from build123d import *

# Parameters (mm, degrees)
F0_W        = 40.3080582619
F0_H        = 5.9715644456
F1_DEPTH    = 537
F3_DEPTH    = 1017
F5_DEPTH    = 5
F6_T1_DEPTH = 716.1336390313


# Not quite as in the source:
# - a fillet or chamfer that OpenCascade refuses, or shapes differently, is made with other operations: its cross-section is extruded or revolved along the edge and cut away or added


with BuildPart() as f1:
    # F0 (on Top) → F1 (new body)
    with BuildSketch(Plane.XY):
        Rectangle(F0_W, F0_H)
    extrude(amount=F1_DEPTH)

    # F2 (on Top) → F3 (join)
    with BuildSketch(Plane.XY):
        Polygon((6.5744029718, -8.407556447), (10.5938451005, -1.2962352533), (8.407556447, 6.5744029718), (1.2962352533, 10.5938451005), (-6.5744029718, 8.407556447), (-10.5938451005, 1.2962352533), (-8.407556447, -6.5744029718), (-1.2962352533, -10.5938451005), align=None)
    extrude(amount=-F3_DEPTH)

    # F4 (on Top) → F5 (join)
    with BuildSketch(Plane.XY):
        Polygon((31.1715127681, -0.1368859226), (15.7043030704, 26.9268789703), (-15.4672096977, 27.0637648929), (-31.1715127681, 0.1368859226), (-15.7043030704, -26.9268789703), (15.4672096977, -27.0637648929), align=None)
    extrude(amount=F5_DEPTH)

    # F6: fillet of radius 270.3919189858 on 1 edges, made by hand

    # F6_s2 → F6_t1 (cut)
    with BuildSketch(Plane.XZ.offset(-358.0668195157)):
        with BuildLine():
            ThreePointArc((-20.1540291309, 537), (9.881896476, 468.7882231999), (20.1540291309, 394.9675850829))
            Line((20.1540291309, 394.9675850829), (20.1540291309, 537))
            Line((20.1540291309, 537), (-20.1540291309, 537))
        make_face()
    extrude(amount=F6_T1_DEPTH, mode=Mode.SUBTRACT)


solid = f1.part
Part model, mm, in its own coordinate system. A direction names the side the tool comes from. Coordinates: 2 decimals unless noted, no trailing zeros. Loops run counter-clockwise (first coordinate to the right, second up) from the corner with the lowest first, then second, coordinate; pieces in that order, holes last. Notation, with made-up numbers: M 24.25,42.25 L 40.25,42.25 A21 cw 40.25,71.25 Z; hole C -19,-29.75 d1. An arc over 180 degrees is marked long. Use a Markdown table: item, result. Add a question column.
Q1. Which spindle directions (+Z, -Z, +X, -X, +Y, -Y) get a long thin tool onto all of the face, cutting with end or side? Do faces 1 (the flat face through (0, -2.986, 267)), 2 (the flat face through (0, 2.986, 267)), 3 (the flat face through (13, 0, 0)). Say none if no direction does.
Q2. Cut at A-A (z = -885). Write the cut outline in (x, y).
Q3. Probe L1, parallel to Z at x = -19, y = 20; L2, parallel to X at y = -1, z = 401.5; L3, parallel to Y at x = 5, z = 178.5. List the from-to ranges inside material, lowest first.
Q4. Pin check, flat tips, straight feed: P1, Ø8, axis at y = 5.5, z = -114, coming from the +X side; P2, Ø8, axis at y = -16, z = -463, coming from the -X side; P3, Ø3, axis at x = 2, y = 18, coming from the +Z side; P4, Ø3, axis at y = -1.5, z = 236.5, coming from the +X side. Stop position of each tip, or through.
Worked out:
| question | item | result |
|---|---|---|
| 1 | face 1 | +Z, +X, -X, -Y |
| 1 | face 2 | +Z, +X, -X, +Y |
| 1 | face 3 | -Z |
| 2 | outline | M -10.59,1.3 L -8.41,-6.57 L -1.3,-10.59 L 6.57,-8.41 L 10.59,-1.3 L 8.41,6.57 L 1.3,10.59 L -6.57,8.41 Z |
| 3 | L1 | z = 0 to 5 |
| 3 | L2 | x = -20.15 to 20.08 |
| 3 | L3 | y = -2.99 to 2.99 |
| 4 | P1 | stops at x = 9.82 |
| 4 | P2 | passes through |
| 4 | P3 | stops at z = 5 |
| 4 | P4 | stops at x = 20.15 |
